Verification items for the finished model (mm, model axes). Face numbers are marked on the shaded views. A direction names the side the tool comes from. Give positions to 0.01 mm unless a question says otherwise; leave off trailing zeros. Loops run counter-clockwise (first coordinate to the right, second up) from the corner with the lowest first, then second, coordinate; pieces in that order, holes last. Notation, with made-up numbers: M 39,87.25 L 50,87.25 A15 ccw 50,105.25 Z; hole C -22.75,73.25 d1. An arc over 180 degrees is marked long. Use CSV: the item, a comma, the result in double quotes.
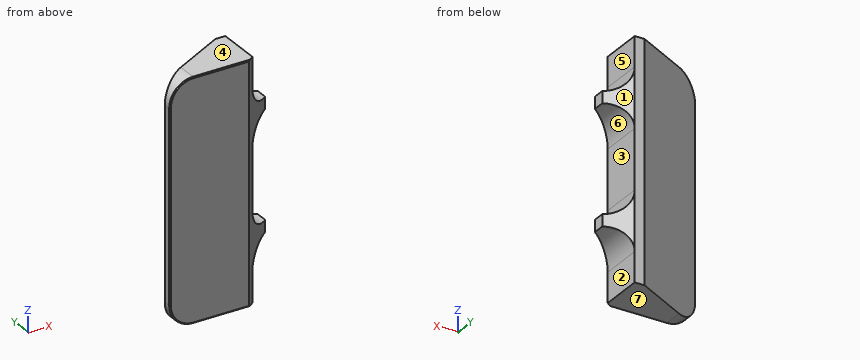
from build123d import *

# Parameters (mm, degrees)
EXTRUDE1_DEPTH     = 60
CUT_EXTRUDE1_DEPTH = 13
FILLET1_R          = 6
CHAMFER1_SIZE      = 0.25


with BuildPart() as part:
    # Sketch1 → Extrude1 (new body)
    with BuildSketch(Plane.XY):
        Polygon((0, 0), (20, 0), (27.5, 5.5), (27.5, 8.5), (21.5, 12), (19, 12), (0, 2), align=None)
    extrude(amount=EXTRUDE1_DEPTH)

    # Sketch2 → Cut-Extrude1 (cut, through all)
    with BuildSketch(Plane(origin=(0, 0, 0), x_dir=(1, 0, 0), z_dir=(0, 1, 0))):
        with BuildLine():
            Line((27.5, -13.5), (27.5, -16.5))
            ThreePointArc((27.5, -16.5), (23.257359313, -18.257359313), (21.5, -22.5))
            Line((21.5, -22.5), (21.5, -37.5))
            ThreePointArc((21.5, -37.5), (23.257359313, -41.742640687), (27.5, -43.5))
            Line((27.5, -43.5), (27.5, -46.5))
            ThreePointArc((27.5, -46.5), (23.257359313, -48.257359313), (21.5, -52.5))
            Line((21.5, -52.5), (21.5, -60))
            Line((21.5, -60), (28.5, -60))
            Line((28.5, -60), (28.5, 0))
            Line((28.5, 0), (21.5, 0))
            Line((21.5, 0), (21.5, -7.5))
            ThreePointArc((21.5, -7.5), (23.257359313, -11.742640687), (27.5, -13.5))
        make_face()
    extrude(amount=CUT_EXTRUDE1_DEPTH, mode=Mode.SUBTRACT)

    # Fillet1
    fillet1_edges = [part.edges().sort_by_distance(p)[0] for p in [
        (0, 1, 60),
        (0, 1, 0),
    ]]
    fillet(fillet1_edges, radius=FILLET1_R)

    # Chamfer1
    chamfer1_edges = [part.edges().sort_by_distance(p)[0] for p in [
        (0, 0, 30),
        (13, 0, 0),
        (13, 0, 60),
        (1.757359313, 0, 58.242640687),
        (1.757359313, 0, 1.757359313),
    ]]
    chamfer(chamfer1_edges, length=CHAMFER1_SIZE)


solid = part.part
(1) Section check B-B on z = 35.5. Record the cut outline in (x, y).
Calculated:
outline,"M 0,0.25 L 0.25,0 L 20,0 L 21.5,1.1 L 21.5,12 L 19,12 L 0,2 Z"
(2) Depth check by flat-ended pin: pin 1 Ø4 at (y, z) = (4.5, 32.5) entering from -X; pin 2 Ø6 at (x, z) = (3, 18) entering from +Y; pin 3 Ø6 at (y, z) = (5, 5) entering from +X. Enter the tip coordinate at first touch or a pass-through.
Calculated:
pin 1,"stops at x = 0.95"
pin 2,"stops at y = 5.16"
pin 3,"stops at x = 21.52"
(3) Section check C-C on x = 14.75. Record the cut outline in (y, z), plus the area to 3 significant figures.
Calculated:
outline,"M 0,0.25 L 0.25,0 L 9.76,0 L 9.76,60 L 0.25,60 L 0,59.75 Z"
area,"586 mm²"
(4) Mould release check, pull along Z, two halves, no side actions. Record for the marked faces 4, 5, 6 and 7: released by +Z, released by -Z, zero draft, split by the parting line, or undercut.
Calculated:
face 4,"released by +Z"
face 5,"zero draft"
face 6,"undercut"
face 7,"released by -Z"
(5) Scan lines: L1, parallel to Z at x = 25.75, y = 8.75; L2, parallel to Z at x = 23, y = 9.75; L3, parallel to Y at x = 13, z = 3. Record each from-to range of solid material in increasing order. Write a range as from..to.
Calculated:
L1,"z = 13.24..16.76, 43.24..46.76"
L2,"z = 11.47..18.53, 41.47..48.53"
L3,"y = 0..8.84"
(6) Section check A-A on y = 6.5. Record the cut outline in (x, z), plus the area to 3 significant figures.
Calculated:
outline,"M 8.55,0 L 21.5,0 L 21.5,7.5 A6 cw 27.5,13.5 L 27.5,16.5 A6 cw 21.5,22.5 L 21.5,37.5 A6 cw 27.5,43.5 L 27.5,46.5 A6 cw 21.5,52.5 L 21.5,60 L 8.55,60 Z"
area,"844 mm²"
(7) Section check D-D on y = 9.5. Record the cut outline in (x, z).
Calculated:
outline,"M 14.25,0 L 21.5,0 L 21.5,7.5 A6 cw 25.79,13.25 L 25.79,16.75 A6 cw 21.5,22.5 L 21.5,37.5 A6 cw 25.79,43.25 L 25.79,46.75 A6 cw 21.5,52.5 L 21.5,60 L 14.25,60 Z"
(8) Tool access check on the marked faces 1, 2 and 3. Record the directions out of +Z, -Z, +X, -X, +Y, -Y that give a thin tool (end or side, any length) a straight path to the whole face; none if there is none.
Calculated:
face 1,"+Z, -Z, +X, +Y"
face 2,"-Z, +X, +Y, -Y"
face 3,"+X, +Y, -Y"
